from build123d import *

# Parameters (mm, degrees)
SKETCH4_W           = 25
SKETCH4_H           = 24.37499982
REVOLVE1_ANGLE      = 45
BOSS_EXTRUDE1_DEPTH = 25
CIRPATTERN1_COUNT   = 25
CIRPATTERN1_ANGLE   = 43.2
SWEEP1_DEPTH        = 6.35
SKETCH18_R          = 2.54
CUT_EXTRUDE1_DEPTH  = 364.676609435
CHAMFER1_SIZE       = 2.0574
CHAMFER1_SIZE2      = 1.788470534


# Read off the part's stored shape, not the designer's step: Sweep1
with BuildPart() as part:
    # Sketch4 → Revolve1 (revolve)
    with BuildSketch(Plane(origin=(0, 0, 0), x_dir=(0, 0, -1), z_dir=(1, 0, 0))):
        with Locations((-12.5, 265.31250009)):
            Rectangle(SKETCH4_W, SKETCH4_H)
    revolve(axis=Axis((0, 0, 25), (0, 0, -1)), revolution_arc=REVOLVE1_ANGLE)

    # Sketch16 → Boss-Extrude1 (add)
    with BuildSketch(Plane(origin=(0, 0, 0), x_dir=(-1, 0, 0), z_dir=(0, 0, -1))):
        with BuildLine():
            ThreePointArc((-3.183813967, 253.104976333), (0, 253.12500018), (3.183813967, 253.104976333))
            ThreePointArc((3.183813967, 253.104976333), (2.085257529, 250.317161386), (1.070720498, 247.497683944))
            ThreePointArc((1.070720498, 247.497683944), (0, 247.5), (-1.070720498, 247.497683944))
            ThreePointArc((-1.070720498, 247.497683944), (-2.085257529, 250.317161386), (-3.183813967, 253.104976333))
        make_face()
    boss_extrude1 = extrude(amount=-BOSS_EXTRUDE1_DEPTH)

    # CirPattern1: Boss-Extrude1 ×25 about axis
    cirpattern1_axis = Axis((0, 0, 0), (0, 0, -1))
    for i in range(1, CIRPATTERN1_COUNT):
        add(boss_extrude1.rotate(cirpattern1_axis, i * CIRPATTERN1_ANGLE / (CIRPATTERN1_COUNT - 1)))

    # Sweep1 outline → Sweep1 (add)
    with BuildSketch(Plane.XY):
        with BuildLine():
            Line((196.222131779, 196.222131779), (209.692515961, 209.692515961))
            ThreePointArc((209.692515961, 209.692515961), (113.484771868, 273.976475366), (0, 296.55))
            Line((0, 296.55), (0, 277.5))
            ThreePointArc((0, 277.5), (106.194652481, 256.376570272), (196.222131779, 196.222131779))
        make_face()
    extrude(amount=SWEEP1_DEPTH)

    # Sketch18 → Cut-Extrude1 (cut, through all)
    with BuildSketch(Plane.XY.offset(6.35)):
        with Locations((25.015877062, 285.93278322)):
            Circle(SKETCH18_R)
        with Locations((82.319697869, 274.966939772)):
            Circle(SKETCH18_R)
        with Locations((136.222171127, 252.639804303)):
            Circle(SKETCH18_R)
        with Locations((184.49611367, 219.873906286)):
            Circle(SKETCH18_R)
    extrude(amount=-CUT_EXTRUDE1_DEPTH, mode=Mode.SUBTRACT)

    # Chamfer1
    chamfer1_edges = [part.edges().sort_by_distance(p)[0] for p in [
        (22.475877062, 285.93278322, 6.35),
        (79.779697869, 274.966939772, 6.35),
        (133.682171127, 252.639804303, 6.35),
        (181.95611367, 219.873906286, 6.35),
    ]]
    chamfer1_side = [part.faces().sort_by_distance(p)[0] for p in [
        (107.078815813, 258.511129376, 6.35),
    ]]
    chamfer(chamfer1_edges, length=CHAMFER1_SIZE, length2=CHAMFER1_SIZE2, reference=chamfer1_side[0])


solid = part.part
Could you check a few things on this model? Use its own coordinates, in mm. A direction names the side the tool comes from. Give positions to 0.01 mm unless a question says otherwise; leave off trailing zeros. Order: outer loops, then holes, each group sorted by start corner. A loop starts at its lowest first (then second) coordinate and runs counter-clockwise, first axis right, second up. Notation, with made-up numbers: (-9.75, -33.5) -> (49.25, -33.5) arc R17 cw to (49.25, -17.5) -> close; hole circle Ø8 at (-15.75, 31.5). An arc over 180 degrees is marked (long way). Return JSON: item names as keys, results as strings.
1. For pin 1 Ø10 at (x, z) = (115, 19.5) entering from +Y; pin 2 Ø3 at (x, z) = (81, 17) entering from +Y; pin 3 Ø5 at (x, z) = (48.5, 7.5) entering from -Y, each with a flat end and sliding along its axis, tell me the tip position at first contact or that it passes through.
Answer list:
{"pin 1": "stops at y = 254.77", "pin 2": "stops at y = 265.87", "pin 3": "stops at y = 242.91"}
2. I need wall thicknesses on line 1 (Z direction, x = 54, y = 285); line 2 (X direction, y = 190.5, z = 11.5); line 3 (X direction, y = 197.5, z = 7.5). Which ranges of each line are inside material? Lowest first, please. Write a range as from..to.
Answer list:
{"line 1": "z = 0..6.35", "line 2": "x = 158.01..159.38, 164.48..190.5", "line 3": "x = 151.28..156.71, 158.32..194.94"}
3. On a 3-axis mill with a long thin cutter (end or side, diameter ignored), from which of +Z, -Z, +X, -X, +Y, -Y can I reach the whole of each face in a straight line? I mean faces 1 (the cylindrical face through (145.457, 203.777, 12.325)), 2 (the cylindrical face through (2.07, 250.28, 12.32)), 3 (the flat face through (0, 270, 10)), 4 (the cylindrical face through (114.99, 273.35, 3.13)). Say none if no direction works.
Answer list:
{"face 1": "+Z, -Z", "face 2": "+Z, -Z, -Y", "face 3": "+Z, -Z, -X, +Y", "face 4": "+Z, -Z, +X, +Y"}
4. Thinking about a two-plate mould opening in Y: for faces 5 (the cylindrical face through (101.298, 228.871, 12.325)), 6 (the cylindrical face through (104.696, 227.423, 12.325)), which applies, pulls with the +Y half, pulls with the -Y half, needs draft (parallel to the pull), parting line crosses it, or undercut?
Answer list:
{"face 5": "pulls with the -Y half", "face 6": "undercut"}
5. Imagine slicing it at A-A on y = 263.5. List the corners of the cut face in (x, z) for me.
Answer list:
{"outline": "(0, 0) -> (136.05, 0) -> (136.05, 6.35) -> (87.03, 6.35) -> (87.03, 25) -> (0, 25) -> close"}
